```python
from build123d import *

# Parameters (mm, degrees)
SKETCH1_W               = 37
SKETCH1_H               = 16
BOSS_EXTRUDE1_DEPTH     = 3
SKETCH2_W               = 2
SKETCH2_H               = 16
BOSS_EXTRUDE2_DEPTH     = 25
FILLET1_R               = 5
CUT_EXTRUDE1_DEPTH      = 46.365184889
CUT_EXTRUDE1_DEPTH_BACK = 46.365184889
SKETCH3_R               = 0.5
BOSS_EXTRUDE3_DEPTH     = 3


with BuildPart() as part:
    # Sketch1 → Boss-Extrude1 (new body)
    with BuildSketch(Plane(origin=(0, 0, 0), x_dir=(1, 0, 0), z_dir=(0, 1, 0))):
        Rectangle(SKETCH1_W, SKETCH1_H)
    extrude(amount=BOSS_EXTRUDE1_DEPTH)

    # Sketch2 → Boss-Extrude2 (add)
    with BuildSketch(Plane.XZ):
        with Locations((17.5, 0)):
            Rectangle(SKETCH2_W, SKETCH2_H)
        with Locations((-17.5, 0)):
            Rectangle(SKETCH2_W, SKETCH2_H)
    extrude(amount=BOSS_EXTRUDE2_DEPTH)

    # Fillet1
    fillet1_edges = [part.edges().sort_by_distance(p)[0] for p in [
        (17.5, -25, 8),
        (17.5, -25, -8),
        (-17.5, -25, -8),
        (-17.5, -25, 8),
    ]]
    fillet(fillet1_edges, radius=FILLET1_R)

    # Sketch3 → Cut-Extrude1 (cut, two sides: drawn at the far end of the back side and taken through both)
    with BuildSketch(Plane(origin=(18.5, 0, 0), x_dir=(0, 0, -1), z_dir=(1, 0, 0)).offset(-CUT_EXTRUDE1_DEPTH_BACK)):
        with Locations((0, -20)):
            Circle(SKETCH3_R)
    extrude(amount=CUT_EXTRUDE1_DEPTH + CUT_EXTRUDE1_DEPTH_BACK, mode=Mode.SUBTRACT)

    # Sketch4 → Boss-Extrude3 (add)
    with BuildSketch(Plane.ZY.offset(18.5)):
        with BuildLine():
            Line((8, 3), (-8, 3))
            add(Edge.make_bspline(
                [(-8, 3), (2.138723357, 62.272306254), (0, 123)],
                knots=[0, 0, 0, 1, 1, 1], degree=2))
            add(Edge.make_bspline(
                [(8, 3), (22.794261884, 63.3166085), (0, 123)],
                knots=[0, 0, 0, 1, 1, 1], degree=2))
        make_face()
    extrude(amount=-BOSS_EXTRUDE3_DEPTH)


solid = part.part
```
The model under review builds one solid part; all positions refer to its coordinate system, in mm. A direction names the side the tool comes from. Give positions to 0.01 mm unless a question says otherwise; leave off trailing zeros. Loops run counter-clockwise (first coordinate to the right, second up) from the corner with the lowest first, then second, coordinate; pieces in that order, holes last. Notation, with made-up numbers: (65, 28) - (110, 28) arc R21 cw to (110, 59) - close; hole circle Ø10 at (26, 29). An arc over 180 degrees is marked (long way). Answer as a JSON object with one key per item and string values.
Q1. Add section A-A on x = 5. State the section outline as (y, z) points, plus the area to 3 significant figures.
Worked out:
{"outline": "(0, -8) - (3, -8) - (3, 8) - (0, 8) - close", "area": "48.0 mm^2"}
Q2. To check wall thickness, follow line 1 along Z through (x, y) = (-17.15, -20); line 2 along Y through (x, z) = (17.1, 0); line 3 along X through (y, z) = (-11, -6.5). State the ranges of each line that lie inside material, in increasing order.
Worked out:
{"line 1": "z = -8 to -0.5, 0.5 to 8", "line 2": "y = -25 to -20.5, -19.5 to 3", "line 3": "x = -18.5 to -16.5, 16.5 to 18.5"}
Q3. Insertion check: pin 1 (2 mm diameter, centred on y = 15, z = -3, fed in from +X); pin 2 (4 mm diameter, centred on x = 10, z = 6, fed in from +Y); pin 3 (8 mm diameter, centred on x = 0, y = -2.5, fed in from +Z). Each pin has a flat end and moves straight along its axis. Give the tip position at first contact, or say it passes through.
Worked out:
{"pin 1": "stops at x = -15.5", "pin 2": "stops at y = 3", "pin 3": "stops at z = 8"}
Q4. For faces 1 (the flat face through (-4, 1, -8)), 2 (the flat face through (1, 3, 0)), 3 (the cylindrical face through (-17, -24, -6)), 4 (the flat face through (0, 0, 0)), 5 (the flat face through (-4, 1, 8)), list the 3-axis set-ups (+Z, -Z, +X, -X, +Y, -Y) from which the entire face can be reached by the end or side of a thin tool; tool diameter is ignored.
Worked out:
{"face 1": "-Z, +X, -X, +Y, -Y", "face 2": "+Z, -Z, +X, +Y", "face 3": "-Z, +X, -X, -Y", "face 4": "+Z, -Z, -Y", "face 5": "+Z, +X, -X, -Y"}
Q5. Mouldability with a two-part tool opening along X and no side actions: class faces 6 (the flat face through (16.5, -12, 0)), 7 (the flat face through (18.5, -11, 0)), 8 (the cylindrical face through (-17, -24, 6)), 9 (the flat face through (-18.5, 34, 4)) as +X half, -X half, draft (parallel to the pull), parting line (faces both ways), or undercut.
Worked out:
{"face 6": "undercut", "face 7": "+X half", "face 8": "draft", "face 9": "-X half"}
